Work out the finished part from the listing and answer in its coordinate system (mm). Round coordinates to 2 decimals unless told otherwise and drop trailing zeros. Order: outer loops, then holes, each group sorted by start corner. A loop starts at its lowest first (then second) coordinate and runs counter-clockwise, first axis right, second up. Notation, with made-up numbers: (-2, 15) - (40, 15) arc R15 ccw to (40, 23) - close; hole circle Ø2 at (46.25, 19). An arc over 180 degrees is marked (long way). Use one line per item in the form item = value. Start each with the question number.
Q1. For a pull along X with two mould halves and no side action, classify faces 1 (the flat face through (-3.449, 6.086, 2.129)), 2 (the cylindrical face through (-3.971, -3.045, 2.891)), 3 (the flat face through (3.546, 6.03, 2.129)) as +X half, -X half, draft (parallel to the pull), parting line (faces both ways), or undercut.
Q2. The part is cut by section C-C on y = 7. Determine the outline of the cut face in (x, z).
Q3. Given P1, Ø1.5, axis at x = -2.5, z = 2.5, coming from the +Y side, flat-ended and moving along its own axis, determine where the tip first touches the part or whether it passes through.
Q4. The part is cut by section B-B on z = 1.75. Determine the outline of the cut face in (x, y), plus the area to 3 significant figures.
Q5. The part is cut by section D-D on z = 4.6. Determine the outline of the cut face in (x, y), plus the area to 3 significant figures.
Q6. Find the intervals of material crossed by line 1 (X direction, y = -2, z = 1.6); line 2 (X direction, y = 1, z = 4.15); line 3 (Y direction, x = 2.75, z = 4.4), in increasing order. Write a range as [from, to].
Q7. The part is cut by section A-A on y = 0. Determine the outline of the cut face in (x, z).
from build123d import *

# Parameters (mm, degrees)
F0_R     = 5.0038
F1_DEPTH = 5.08
F2_SIZE  = 0.762
F3_SIZE  = 0.762


with BuildPart() as f1:
    # F0 (on Top) → F1 (new body)
    with BuildSketch(Plane.XY):
        Polygon((0, 8.0772), (-6.99506, 4.0386), (-6.99506, -4.0386), (0, -8.0772), (6.99506, -4.0386), (6.99506, 4.0386), align=None)
        Circle(F0_R, mode=Mode.SUBTRACT)
    extrude(amount=F1_DEPTH)

    # F2
    f2_edges = [f1.edges().sort_by_distance(p)[0] for p in [
        (-3.49753, 6.0579, 5.08),
        (-6.99506, 0, 5.08),
        (-3.49753, -6.0579, 5.08),
        (3.49753, -6.0579, 5.08),
        (6.99506, 0, 5.08),
        (3.49753, 6.0579, 5.08),
    ]]
    chamfer(f2_edges, length=F2_SIZE)

    # F3
    f3_edges = [f1.edges().sort_by_distance(p)[0] for p in [
        (-5.0038, 0, 0),
    ]]
    chamfer(f3_edges, length=F3_SIZE)


solid = f1.part
Found:
q1.face_1 = -X half
q1.face_2 = undercut
q1.face_3 = +X half
q2.outline = (-1.87, 0) - (1.87, 0) - (1.87, 4.32) - (0.34, 5.08) - (-0.34, 5.08) - (-1.87, 4.32) - close
q3.P1 = 7.07
q4.outline = (-7, -4.04) - (0, -8.08) - (7, -4.04) - (7, 4.04) - (0, 8.08) - (-7, 4.04) - close; hole circle Ø10.01 at (0, 0)
q4.area = 90.8 mm²
q5.outline = (-6.71, -3.88) - (0, -7.75) - (6.71, -3.88) - (6.71, 3.88) - (0, 7.75) - (-6.71, 3.88) - close; hole circle Ø10.01 at (0, 0)
q5.area = 77.5 mm²
q6.line_1 = [-7, -4.59], [4.59, 7]
q6.line_2 = [-7, -4.9], [4.9, 7]
q6.line_3 = [-6.39, -4.18], [4.18, 6.39]
q7.outline = (-7, 0) - (-5.77, 0) - (-5, 0.76) - (-5, 5.08) - (-6.23, 5.08) - (-7, 4.32) - close; (5, 0.76) - (5.77, 0) - (7, 0) - (7, 4.32) - (6.23, 5.08) - (5, 5.08) - close
